Design review of the part built by this model. Coordinates are the model's own, in mm. Give positions to 0.01 mm unless a question says otherwise; leave off trailing zeros. Order: outer loops, then holes, each group sorted by start corner. A loop starts at its lowest first (then second) coordinate and runs counter-clockwise, first axis right, second up. Notation, with made-up numbers: M 74.25,87.25 L 80.25,87.25 A13 ccw 80.25,108.25 Z; hole C 85,14 d3. An arc over 180 degrees is marked long. Answer as a JSON object with one key per item and string values.
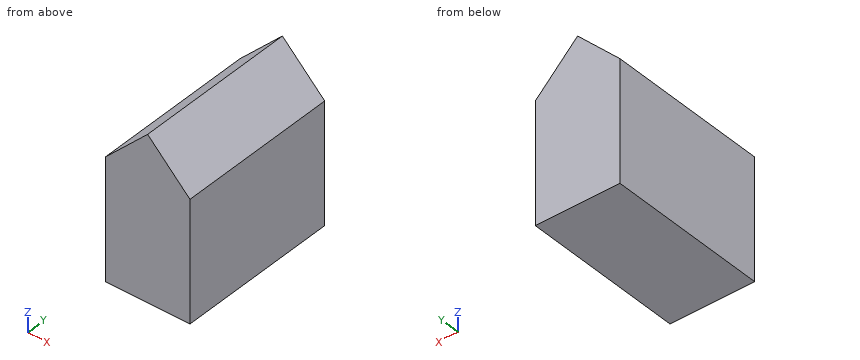
from build123d import *

# Parameters (mm, degrees)
F0_W     = 13
F0_H     = 18.5
F1_DEPTH = 12.5


with BuildPart() as f1:
    # F0 (on Front) → F1 (new body, symmetric)
    with BuildSketch(Plane.XZ):
        with Locations((0, 9.25)):
            Rectangle(F0_W, F0_H)
        Polygon((0, 25), (-6.5, 18.5), (6.5, 18.5), align=None)
    extrude(amount=F1_DEPTH, both=True)


solid = f1.part
(1) To check wall thickness, follow L1, parallel to Z at x = 1.75, y = 10.75; L2, parallel to Z at x = -0.5, y = 4.5; L3, parallel to X at y = 8, z = 19.5. State the ranges of each line that lie inside material, in increasing order. Write a range as from..to.
Checked values:
{"L1": "z = 0..23.25", "L2": "z = 0..24.5", "L3": "x = -5.5..5.5"}
(2) Insertion check: pin 1 (1.5 mm diameter, centred on x = 0, y = -1.5, fed in from +Z); pin 2 (6 mm diameter, centred on y = 3, z = 22.5, fed in from +X); pin 3 (6 mm diameter, centred on x = -5, y = 2.5, fed in from +Z). Each pin has a flat end and moves straight along its axis. Give the tip position at first contact, or say it passes through.
Checked values:
{"pin 1": "stops at z = 25", "pin 2": "stops at x = 5.5", "pin 3": "stops at z = 23"}
(3) We need section B-B (y = -8.75). Write out the cut boundary in (x, z).
Checked values:
{"outline": "M -6.5,0 L 6.5,0 L 6.5,18.5 L 0,25 L -6.5,18.5 Z"}
(4) We need section A-A (x = -1.25). Write out the cut boundary in (y, z).
Checked values:
{"outline": "M -12.5,0 L 12.5,0 L 12.5,23.75 L -12.5,23.75 Z"}
(5) We need section C-C (z = 21.75). Write out the cut boundary in (x, y), plus the area to 4 significant figures.
Checked values:
{"outline": "M -3.25,-12.5 L 3.25,-12.5 L 3.25,12.5 L -3.25,12.5 Z", "area": "162.5 mm^2"}
